Read the model definition and answer for the solid it produces. Units are mm, in the model's axes. Face numbers are marked on the shaded views. A direction names the side the tool comes from. Round coordinates to 2 decimals unless told otherwise and drop trailing zeros. Order: outer loops, then holes, each group sorted by start corner. A loop starts at its lowest first (then second) coordinate and runs counter-clockwise, first axis right, second up. Notation, with made-up numbers: (-26, 24.25) -> (-17, 24.25) arc R11 cw to (-17, 43.25) -> close; hole circle Ø10 at (30, 33.5). An arc over 180 degrees is marked (long way). Use a Markdown table: item, result. Add a question column.
1. Section D-D, the plane z = 0.5 is taken. Give the vertices of the cut face in (x, y), then the cut area to 3 significant figures.
2. Section C-C, the plane y = 8.5 is taken. Give the vertices of the cut face in (x, z), then the cut area to 3 significant figures.
3. Section A-A, the plane y = 2.25 is taken. Give the vertices of the cut face in (x, z), then the cut area to 3 significant figures.
4. Consider L1, parallel to X at y = 1.95, z = 0; L2, parallel to Y at x = -8.8, z = 0; L3, parallel to Y at x = 9, z = -1. Determine where each line is inside the solid, lowest interval first. Write a range as [from, to].
5. Section B-B, the plane x = 0 is taken. Give the vertices of the cut face in (y, z).
6. For the marked faces 5 and 6, determine the directions among +Z, -Z, +X, -X, +Y, -Y from which every point of the face is accessible in a straight line to the end or side of a thin tool.
7. The mould has two halves that part along Z. Classify the marked faces 1, 2, 3 and 4: +Z half, -Z half, draft (parallel to the pull), parting line (faces both ways), or undercut.
8. Given pin 1 (5 mm diameter, centred on y = 17, z = -3, fed in from +X); pin 2 (8 mm diameter, centred on x = -1, y = 4, fed in from -Z); pin 3 (5 mm diameter, centred on x = -2.5, z = -2, fed in from +Y), each flat-ended and moving along its own axis, determine where each tip first touches the part or whether it passes through.
```python
from build123d import *

# Parameters (mm, degrees)
SKETCH_1_W          = 20
SKETCH_1_H          = 20
EXTRUDE_1_DEPTH     = 20
SKETCH_2_W          = 17
SKETCH_2_H          = 17
CUT_EXTRUDE_1_DEPTH = 20
FILLET_1_R          = 10
SKETCH_3_R          = 2.5
CUT_EXTRUDE_2_DEPTH = 20
SKETCH_4_R          = 3
CUT_EXTRUDE_3_DEPTH = 20


with BuildPart() as part:
    # 草图1 → 凸台-拉伸1 (new body)
    with BuildSketch(Plane(origin=(0, 0, 0), x_dir=(1, 0, 0), z_dir=(0, 1, 0))):
        Rectangle(SKETCH_1_W, SKETCH_1_H)
    extrude(amount=EXTRUDE_1_DEPTH)

    # 草图2 → 切除-拉伸1 (cut)
    with BuildSketch(Plane.XY.offset(10)):
        with Locations((1.5, 11.5)):
            Rectangle(SKETCH_2_W, SKETCH_2_H)
    extrude(amount=-CUT_EXTRUDE_1_DEPTH, mode=Mode.SUBTRACT)

    # 圆角1
    fillet_1_edges = [part.edges().sort_by_distance(p)[0] for p in [
        (-8.5, 20, -10),
        (-8.5, 20, 10),
    ]]
    fillet(fillet_1_edges, radius=FILLET_1_R - 0.0001)  # a hair under: the kernel refuses the full size

    # 草图3 → 切除-拉伸2 (cut)
    with BuildSketch(Plane(origin=(-7, 0, 0), x_dir=(0, 0, -1), z_dir=(1, 0, 0))):
        with Locations((0, 10)):
            Circle(SKETCH_3_R)
    extrude(amount=-CUT_EXTRUDE_2_DEPTH, mode=Mode.SUBTRACT)

    # 草图4 → 切除-拉伸3 (cut)
    with BuildSketch(Plane(origin=(0, 3, 0), x_dir=(1, 0, 0), z_dir=(0, 1, 0))):
        with Locations(Location((0, 0, 0), (0, 0, 270))):
            Circle(SKETCH_4_R)
    extrude(amount=-CUT_EXTRUDE_3_DEPTH, mode=Mode.SUBTRACT)


solid = part.part
```
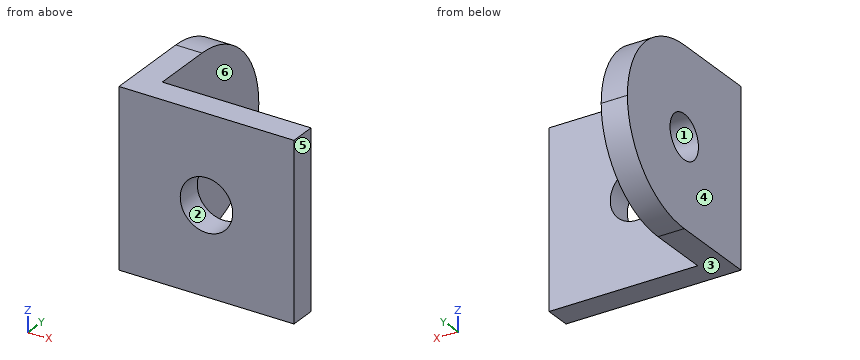
Verdict:
| question | item | result |
|---|---|---|
| 1 | outline | (-10, 0) -> (-2.96, 0) -> (-2.96, 3) -> (-7, 3) -> (-7, 7.55) -> (-10, 7.55) -> close; (-10, 12.45) -> (-7, 12.45) -> (-7, 19.99) -> (-10, 19.99) -> close; (2.96, 0) -> (10, 0) -> (10, 3) -> (2.96, 3) -> close |
| 1 | area | 78.5 mm2 |
| 2 | outline | (-10, -10) -> (-7, -10) -> (-7, -2) -> (-10, -2) -> close; (-10, 2) -> (-7, 2) -> (-7, 10) -> (-10, 10) -> close |
| 2 | area | 48.0 mm2 |
| 3 | outline | (-10, -10) -> (10, -10) -> (10, 10) -> (-10, 10) -> close; hole circle Ø6 at (0, 0) |
| 3 | area | 372 mm2 |
| 4 | L1 | x = [-10, -3], [3, 10] |
| 4 | L2 | y = [0, 7.5], [12.5, 20] |
| 4 | L3 | y = [0, 3] |
| 5 | outline | (0, -10) -> (3, -10) -> (3, -3) -> (0, -3) -> close; (0, 3) -> (3, 3) -> (3, 10) -> (0, 10) -> close |
| 6 | face 5 | +Z, -Z, +X, +Y, -Y |
| 6 | face 6 | +Z, -Z, +X, +Y |
| 7 | face 1 | undercut |
| 7 | face 2 | undercut |
| 7 | face 3 | -Z half |
| 7 | face 4 | draft |
| 8 | pin 1 | stops at x = -7 |
| 8 | pin 2 | stops at z = -10 |
| 8 | pin 3 | stops at y = 3 |
